from build123d import *

# Parameters (mm, degrees)
SKETCH_1_W           = 62.126713746
SKETCH_1_H           = 62.126713746
EXTRUDE_1_DEPTH      = 57
SKETCH_3_W           = 58.126713746
SKETCH_3_H           = 62.126713746
CUT_EXTRUDE_5_DEPTH  = 54
SKETCH_4_W           = 2
SKETCH_4_H           = 62.126713746
EXTRUDE_2_DEPTH      = 24
SKETCH_5_W           = 2
SKETCH_5_H           = 62.126713746
EXTRUDE_3_DEPTH      = 24
SKETCH_6_R           = 1.5
CUT_EXTRUDE_6_DEPTH  = 24
SKETCH_7_R           = 1.5
CUT_EXTRUDE_7_DEPTH  = 24
FILLET_3_R           = 2
FILLET_4_R           = 2
FILLET_5_R           = 2
FILLET_6_R           = 2
SKETCH_1_2_W         = 62.126713746
SKETCH_1_2_H         = 62.126713746
EXTRUDE_4_DEPTH      = 30.59
CUT_EXTRUDE_8_DEPTH  = 70
SKETCH_12_R          = 1.5
CUT_EXTRUDE_9_DEPTH  = 10
CUT_EXTRUDE_10_REACH = 108.26
SKETCH_15_W          = 58.126713746
SKETCH_15_H          = 22.559791582
CUT_EXTRUDE_11_DEPTH = 2
FILLET_7_R           = 2
FILLET_8_R           = 2


with BuildPart() as part:
    # 草图1 → 凸台-拉伸1 (new body)
    with BuildSketch(Plane.XY):
        Rectangle(SKETCH_1_W, SKETCH_1_H)
    extrude(amount=EXTRUDE_1_DEPTH)

    # 草图3 → 切除-拉伸5 (cut)
    with BuildSketch(Plane.XY.offset(57)):
        Rectangle(SKETCH_3_W, SKETCH_3_H)
    extrude(amount=-CUT_EXTRUDE_5_DEPTH, mode=Mode.SUBTRACT)

    # 草图4 → 凸台-拉伸2 (add)
    with BuildSketch(Plane(origin=(31.063356873, 0, 0), x_dir=(0, 0, -1), z_dir=(1, 0, 0))):
        with Locations((-56, 0)):
            Rectangle(SKETCH_4_W, SKETCH_4_H)
    extrude(amount=EXTRUDE_2_DEPTH)

    # 草图5 → 凸台-拉伸3 (add)
    with BuildSketch(Plane.ZY.offset(31.063356873)):
        with Locations((56, 0)):
            Rectangle(SKETCH_5_W, SKETCH_5_H)
    extrude(amount=EXTRUDE_3_DEPTH)

    # 草图6 → 切除-拉伸6 (cut)
    with BuildSketch(Plane.XY.offset(57)):
        with Locations((39.063356873, 12.063356873)):
            Circle(SKETCH_6_R)
        with Locations(Location((-39.063356873, 12.063356873, 0), (0, 0, 270))):
            Circle(SKETCH_6_R)
        with Locations(Location((39.063356873, -12.063356873, 0), (0, 0, 270))):
            Circle(SKETCH_6_R)
        with Locations((-39.063356873, -12.063356873)):
            Circle(SKETCH_6_R)
    extrude(amount=-CUT_EXTRUDE_6_DEPTH, mode=Mode.SUBTRACT)

    # 草图7 → 切除-拉伸7 (cut)
    with BuildSketch(Plane(origin=(0, 0, 0), x_dir=(-1, 0, 0), z_dir=(0, 0, -1))):
        with Locations((-18, 24)):
            Circle(SKETCH_7_R)
        with Locations((18, 24)):
            Circle(SKETCH_7_R)
        with Locations((18, -24)):
            Circle(SKETCH_7_R)
        with Locations((-18, -24)):
            Circle(SKETCH_7_R)
    extrude(amount=-CUT_EXTRUDE_7_DEPTH, mode=Mode.SUBTRACT)

    # 圆角3
    fillet_3_edges = [part.edges().sort_by_distance(p)[0] for p in [
        (55.063356873, -31.063356873, 56),
    ]]
    fillet(fillet_3_edges, radius=FILLET_3_R)

    # 圆角4
    fillet_4_edges = [part.edges().sort_by_distance(p)[0] for p in [
        (55.063356873, 31.063356873, 56),
    ]]
    fillet(fillet_4_edges, radius=FILLET_4_R)

    # 圆角5
    fillet_5_edges = [part.edges().sort_by_distance(p)[0] for p in [
        (-55.063356873, -31.063356873, 56),
    ]]
    fillet(fillet_5_edges, radius=FILLET_5_R)

    # 圆角6
    fillet_6_edges = [part.edges().sort_by_distance(p)[0] for p in [
        (-55.063356873, 31.063356873, 56),
    ]]
    fillet(fillet_6_edges, radius=FILLET_6_R)

    # 草图1<2> → 凸台-拉伸4 (add)
    with BuildSketch(Plane.XY):
        Rectangle(SKETCH_1_2_W, SKETCH_1_2_H)
    extrude(amount=-EXTRUDE_4_DEPTH)

    # 草图11 → 切除-拉伸8 (cut)
    with BuildSketch(Plane(origin=(31.063356873, 0, 0), x_dir=(0, 0, -1), z_dir=(1, 0, 0))):
        Polygon((30.59, 31.063356873), (0, -31.256692995), (30.59, -31.063356873), align=None)
    extrude(amount=-CUT_EXTRUDE_8_DEPTH, mode=Mode.SUBTRACT)

    # 草图12 → 切除-拉伸9 (cut)
    with BuildSketch(Plane(origin=(0, -6.068714237, -12.363601631), x_dir=(-1, 0, 0), z_dir=(0, -0.440632808345781, -0.8976874334696406))):
        with Locations(Location((18, -17.761485842, 0), (0, 0, 90))):
            Circle(SKETCH_12_R)
        with Locations(Location((-18, -17.761485842, 0), (0, 0, 270))):
            Circle(SKETCH_12_R)
        with Locations(Location((18, 30.238514158, 0), (0, 0, 90))):
            Circle(SKETCH_12_R)
        with Locations(Location((-18, 30.238514158, 0), (0, 0, 270))):
            Circle(SKETCH_12_R)
    extrude(amount=-CUT_EXTRUDE_9_DEPTH, mode=Mode.SUBTRACT)

    # 切除-拉伸10: up to this face of the body (flat: up to its plane)
    cut_extrude_10_end = Plane(part.part.faces().sort_by_distance((-29.063356873, 0, 30))[0])
    # 草图14 → 切除-拉伸10 (cut, up to the picked face)
    with BuildSketch(Plane.ZY.offset(-29.063356873), mode=Mode.PRIVATE) as cut_extrude_10_sk1:
        Polygon((3, -29.063356873), (3, 29.063356873), (-27.380346496, 29.063356873), (1.151340775, -29.063356873), align=None)
    cut_extrude_10_tool1 = split(extrude(cut_extrude_10_sk1.sketch, amount=CUT_EXTRUDE_10_REACH, mode=Mode.PRIVATE), bisect_by=cut_extrude_10_end, keep=Keep.BOTH, mode=Mode.PRIVATE)
    add(cut_extrude_10_tool1.solids().sort_by(Axis((29.063357, 8.576401, -7.162129), (-1, 0, 0)))[0], mode=Mode.SUBTRACT)

    # 草图15 → 切除-拉伸11 (cut)
    with BuildSketch(Plane(origin=(0, 31.063356873, 0), x_dir=(1, 0, 0), z_dir=(0, 1, 0))):
        with Locations((0, 14.310104209)):
            Rectangle(SKETCH_15_W, SKETCH_15_H)
    extrude(amount=-CUT_EXTRUDE_11_DEPTH, mode=Mode.SUBTRACT)

    # 圆角7
    fillet_7_edges = [part.edges().sort_by_distance(p)[0] for p in [
        (-31.063356873, 0, -15.342449833),
    ]]
    fillet(fillet_7_edges, radius=FILLET_7_R)

    # 圆角8
    fillet_8_edges = [part.edges().sort_by_distance(p)[0] for p in [
        (31.063356873, 0, -15.342449833),
    ]]
    fillet(fillet_8_edges, radius=FILLET_8_R)


solid = part.part
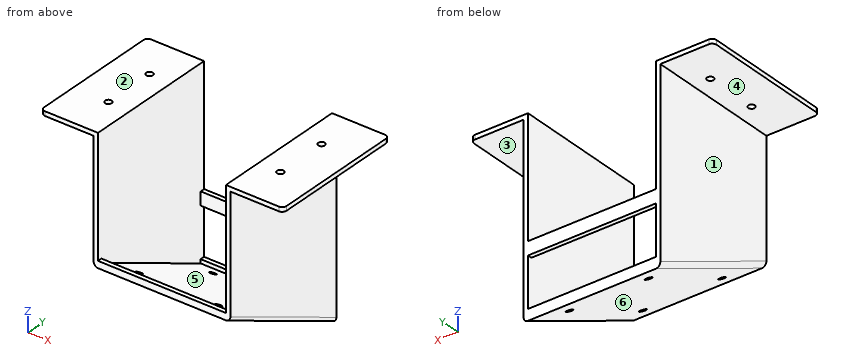
Can you work these out from the model? Positions are in its coordinate system, mm. Face numbers are marked on the shaded views. A direction names the side the tool comes from. Give positions to 0.01 mm unless a question says otherwise; leave off trailing zeros. Order: outer loops, then holes, each group sorted by start corner. A loop starts at its lowest first (then second) coordinate and runs counter-clockwise, first axis right, second up. Notation, with made-up numbers: (64.25, 88) - (122.25, 88) arc R25 ccw to (122.25, 126) - close; hole circle Ø10 at (88, 61.25). An arc over 180 degrees is marked (long way). Write each question's results on one line, items separated by ' | '.
1) Suppose I cut it at C-C, the plane x = -44.5. Write out the boundary of the cut face in (y, z).
Final values:
outline: (-31.06, 55) - (31.06, 55) - (31.06, 57) - (-31.06, 57) - close
2) Suppose I cut it at B-B, the plane z = 48. Write out the boundary of the cut face in (x, y), then the cut area to 3 significant figures.
Final values:
outline: (-31.06, -31.06) - (-29.06, -31.06) - (-29.06, 31.06) - (-31.06, 31.06) - close; (29.06, -31.06) - (31.06, -31.06) - (31.06, 31.06) - (29.06, 31.06) - close | area: 249 mm^2
3) On a 3-axis mill with a long thin cutter (end or side, diameter ignored), from which of +Z, -Z, +X, -X, +Y, -Y can I reach the whole of each face in a straight line? I mean the marked faces 1, 2 and 3. Say none if no direction works.
Final values:
face 1: -Z, -X, +Y, -Y | face 2: +Z, +X, -X, +Y, -Y | face 3: -Z, +X, +Y, -Y
4) Suppose I cut it at A-A, the plane x = -21. Write out the boundary of the cut face in (y, z).
Final values:
outline: (-31.06, -0.09) - (31.06, -30.59) - (31.06, -25.59) - (29.06, -25.59) - (29.06, -27.38) - (-29.06, 1.15) - (-29.06, 3) - (-31.06, 3) - close; (29.06, -3.03) - (31.06, -3.03) - (31.06, 3) - (29.06, 3) - close
5) I'm going to push flat-ended pins straight in: pin 1 Ø3 at (y, z) = (-14.5, -8) entering from +X; pin 2 Ø12 at (x, y) = (40, -13) entering from -Z; pin 3 Ø2.5 at (x, y) = (-39.06, -12.06) entering from +Z; pin 4 Ø5 at (x, y) = (30, 4.5) entering from -Z. Where does each tip first touch, or does it pass through?
Final values:
pin 1: stops at x = 31.04 | pin 2: stops at z = 55 | pin 3: passes through | pin 4: stops at z = -18.71
6) Please list where these lines run through material, in increasing order: line 1 along X through (y, z) = (-12, 44.5); line 2 along Z through (x, y) = (-35, 26); line 3 along Y through (x, z) = (-22, -21). Write a range as [from, to].
Final values:
line 1: x = [-31.06, -29.06], [29.06, 31.06] | line 2: z = [55, 57] | line 3: y = [11.53, 16.06]
7) If we mould it in two halves opening along Y, with no side actions, what happens to the marked faces 4, 5 and 6? For each: pulls with the +Y half, pulls with the -Y half, needs draft (parallel to the pull), parting line crosses it, or undercut.
Final values:
face 4: needs draft | face 5: undercut | face 6: pulls with the -Y half
